from build123d import *
from build123d import SkipClean  # not in build123d's __all__

# Parameters (mm, degrees)
F0_W        = 50
F0_H        = 50
F0_R        = 12.5
F1_DEPTH    = 30
F2_DEPTH    = 25
F4_DEPTH    = 25
F6_DEPTH    = 50
F8_DEPTH    = 25
F9_T1_DEPTH = 9.1191559928
F9_T3_DEPTH = 9.1191559928
F9_T5_DEPTH = 9.1191559928
F9_T7_DEPTH = 9.1191559928
F9_T9_DEPTH = 9.1191559928
F10_R       = 2


# Not quite as in the source:
# - a fillet or chamfer that OpenCascade refuses, or shapes differently, is made with other operations: its cross-section is extruded or revolved along the edge and cut away or added
# - after a boolean that leaves OpenCascade's solid faulty, fix() repairs it


with BuildPart() as f1:
    # F0 (on Front) → F1 (new body)
    with BuildSketch(Plane.XZ):
        Rectangle(F0_W, F0_H)
        Circle(F0_R, mode=Mode.SUBTRACT)
    extrude(amount=F1_DEPTH)

    # F0 (on Front) → F2 (join)
    with BuildSketch(Plane.XZ):
        Rectangle(F0_W, F0_H)
        Circle(F0_R, mode=Mode.SUBTRACT)
    extrude(amount=F2_DEPTH)

    # F3 (on face) → F4 (join)
    with BuildSketch(Plane.XZ.offset(30)):
        with BuildLine():
            Line((-8.8388347648, -8.8388347648), (-25, -25))
            Line((-25, -25), (25, -25))
            Line((25, -25), (25, 25))
            Line((25, 25), (8.8388347648, 8.8388347648))
            ThreePointArc((8.8388347648, 8.8388347648), (8.8388347648, -8.8388347648), (-8.8388347648, -8.8388347648))
        make_face()
    with SkipClean():  # cleaning this boolean's faces spoils the solid; the shape is the same uncleaned
        extrude(amount=F4_DEPTH)

    # F5 (on face) → F6 (cut)
    with BuildSketch(Plane(origin=(0, 0, 0), x_dir=(0.7071067812, 0, 0.7071067812), z_dir=(-0.7071067812, 0, 0.7071067812))):
        Polygon((-23.9276695297, -31), (-34.3199743751, -49), (-13.5353646843, -49), align=None)
        Polygon((19.249809042, -35.5263909924), (14.8302387921, -42.8186887872), (18.9357688095, -50.2922977948), (27.4608690767, -50.4736090076), (31.8804393265, -43.1813112128), (27.7749093092, -35.7077022052), align=None)
    extrude(amount=-F6_DEPTH, mode=Mode.SUBTRACT)

    add(f1.part.fix(), mode=Mode.REPLACE)

    # F7 (on face) → F8 (join)
    with BuildSketch(Plane.XZ.offset(30)):
        Polygon((-19.0595779964, 11.4327062681), (-14.9404220036, 11.4327062681), (-12.8808440072, 15), (-14.9404220036, 18.5672937319), (-19.0595779964, 18.5672937319), (-21.1191559928, 15), align=None)
    extrude(amount=F8_DEPTH)

    # F9: fillet of radius 1 on 6 edges, made by hand

    # F9_s2 → F9_t1 (cut)
    with BuildSketch(Plane(origin=(4.5249795266, 0, 7.8374944433), x_dir=(0, 1, 0), z_dir=(-0.5, 0, -0.8660254038))):
        with BuildLine():
            add(Edge.make_bspline(
                [(-54, -25.7897255963), (-55, -25.7897255963), (-55, -24.7897255963)],
                knots=[0, 0, 0, 1, 1, 1], degree=2, weights=[1, 1, 1]))
            Line((-55, -24.7897255963), (-55, -25.7897255963))
            Line((-55, -25.7897255963), (-54, -25.7897255963))
        make_face()
    extrude(amount=F9_T1_DEPTH, mode=Mode.SUBTRACT)

    # F9_s4 → F9_t3 (cut)
    with BuildSketch(Plane(origin=(-13.0249795266, 0, 22.5599263076), x_dir=(0, 1, 0), z_dir=(0.5, 0, -0.8660254038))):
        with BuildLine():
            add(Edge.make_bspline(
                [(-54, -10.7897255963), (-55, -10.7897255963), (-55, -9.7897255963)],
                knots=[0, 0, 0, 1, 1, 1], degree=2, weights=[1, 1, 1]))
            Line((-55, -9.7897255963), (-55, -10.7897255963))
            Line((-55, -10.7897255963), (-54, -10.7897255963))
        make_face()
    extrude(amount=F9_T3_DEPTH, mode=Mode.SUBTRACT)

    # F9_s6 → F9_t5 (cut)
    with BuildSketch(Plane.YZ.offset(-21.5595779964)):
        with BuildLine():
            add(Edge.make_bspline(
                [(-54, 11.4327062681), (-55, 11.4327062681), (-55, 12.4327062681)],
                knots=[0, 0, 0, 1, 1, 1], degree=2, weights=[1, 1, 1]))
            Line((-55, 12.4327062681), (-55, 11.4327062681))
            Line((-55, 11.4327062681), (-54, 11.4327062681))
        make_face()
        with BuildLine():
            add(Edge.make_bspline(
                [(-54, 18.5672937319), (-55, 18.5672937319), (-55, 17.5672937319)],
                knots=[0, 0, 0, 1, 1, 1], degree=2, weights=[1, 1, 1]))
            Line((-55, 17.5672937319), (-55, 18.5672937319))
            Line((-55, 18.5672937319), (-54, 18.5672937319))
        make_face()
    extrude(amount=F9_T5_DEPTH, mode=Mode.SUBTRACT)

    # F9_s8 → F9_t7 (cut)
    with BuildSketch(Plane(origin=(-0.0345984698, 0, -0.0599263076), x_dir=(0, 1, 0), z_dir=(0.5, 0, 0.8660254038))):
        with BuildLine():
            add(Edge.make_bspline(
                [(-54, 18.6551381324), (-55, 18.6551381324), (-55, 19.6551381324)],
                knots=[0, 0, 0, 1, 1, 1], degree=2, weights=[1, 1, 1]))
            Line((-55, 19.6551381324), (-55, 18.6551381324))
            Line((-55, 18.6551381324), (-54, 18.6551381324))
        make_face()
    extrude(amount=F9_T7_DEPTH, mode=Mode.SUBTRACT)

    # F9_s10 → F9_t9 (cut)
    with BuildSketch(Plane(origin=(-8.4654015302, 0, 14.6625055567), x_dir=(0, 1, 0), z_dir=(-0.5, 0, 0.8660254038))):
        with BuildLine():
            add(Edge.make_bspline(
                [(-54, 3.6551381324), (-55, 3.6551381324), (-55, 4.6551381324)],
                knots=[0, 0, 0, 1, 1, 1], degree=2, weights=[1, 1, 1]))
            Line((-55, 4.6551381324), (-55, 3.6551381324))
            Line((-55, 3.6551381324), (-54, 3.6551381324))
        make_face()
    extrude(amount=F9_T9_DEPTH, mode=Mode.SUBTRACT)

    # F10
    f10_edges = [f1.edges().sort_by_distance(p)[0] for p in [
        (25, 0, 0),
        (0, 0, -25),
        (-25, 0, 0),
        (0, 0, 25),
    ]]
    fillet(f10_edges, radius=F10_R)


solid = f1.part
Could you check a few things on this model? Use its own coordinates, in mm. A direction names the side the tool comes from. Give positions to 0.01 mm unless a question says otherwise; leave off trailing zeros. Order: outer loops, then holes, each group sorted by start corner. A loop starts at its lowest first (then second) coordinate and runs counter-clockwise, first axis right, second up.
Item 1: If we section it at D-D, the plane y = -25: Write out the boundary of the cut face in (x, z).
Item 2: If we section it at B-B, the plane y = -34: Write out the boundary of the cut face in (x, z).
Item 3: I'm going to push a flat-ended pin straight in: pin 1 (4.5 mm diameter, centred on x = -16, y = -37.5, fed in from +Z). Where does the tip first touch, or does it pass through?
Item 4: If we section it at C-C, the plane x = 0.5: Write out the boundary of the cut face in (y, z).
Item 5: If we section it at A-A, the plane z = -3: Write out the boundary of the cut face in (x, y), plus the area to 3 significant figures.
Item 6: For faces 1 (the face through (25, -28, 0)), 2 (the face through (22.84, -38.67, 18.74)), 3 (the face through (-20.075, -41.832, 16.809)), 4 (the face through (-17, -42, 11.433)), 5 (the face through (-5.9, -30, 11.5)), which set-ups out of +Z, -Z, +X, -X, +Y, -Y let a thin tool reach every point of the face, with its end or its side?
Item 7: I need wall thicknesses on line 1 (X direction, y = -11.5, z = 0); line 2 (Y direction, x = -19, z = -11.5); line 3 (Y direction, x = -12, z = -19). Which ranges of each line are inside material? Lowest first, please.
Item 8: If we mould it in two halves opening along X, with no side actions, what happens to faces 6 (the face through (22.4, -42.3, 22.4)), 7 (the face through (-13.925, -41.832, 13.191)), 8 (the face through (-17, -42, 18.567)), 9 (the face through (-25, -16, 0))? For each: pulls with the +X half, pulls with the -X half, needs draft (parallel to the pull), parting line crosses it, or undercut.
Values:
1. outline: (-25, -25) - (25, -25) - (25, 25) - (-25, 25) - close; hole circle Ø25 at (0, 0)
2. outline: (-25, -25) - (-11.29, -25) - (-18.14, -18.14) - close; (-21.12, 15) - (-19.06, 11.43) - (-14.94, 11.43) - (-12.88, 15) - (-14.94, 18.57) - (-19.06, 18.57) - close; (-15.69, -15.69) - (-6.39, -25) - (25, -25) - (25, 25) - (8.84, 8.84) arc R12.5 cw to (-8.84, -8.84) - close
3. pin 1: stops at z = 18.57
4. outline: (-55, -25) - (-49, -25) - (-49, -19.64) - (-42.44, -25) - (-2, -25) arc R2 ccw to (0, -23) - (0, -12.49) - (-55, -12.49) - close; (-30, 12.49) - (0, 12.49) - (0, 23) arc R2 ccw to (-2, 25) - (-30, 25) - close
5. outline: (-25, -30) - (-12.13, -30) - (-12.13, 0) - (-23, 0) arc R2 ccw to (-25, -2) - close; (12.13, -55) - (25, -55) - (25, -44.14) - (23.97, -42.82) - (25, -41.62) - (25, -2) arc R2 ccw to (23, 0) - (12.13, 0) - close
5. area: 1,090 mm2
6. face 1: +Z, -Z, +X, +Y, -Y
6. face 2: none
6. face 3: +Z, -X, -Y
6. face 4: -X, -Y
6. face 5: -Y
7. line 1: x = -25 to -12.5, 12.5 to 25
7. line 2: y = -30 to 0
7. line 3: y = -55 to -49, -34.48 to 0
8. face 6: undercut
8. face 7: undercut
8. face 8: needs draft
8. face 9: pulls with the -X half
